CAD build for the part. Positions are in the model's coordinates, mm. A direction names the side the tool comes from. Give positions to 0.01 mm unless a question says otherwise; leave off trailing zeros. Order: outer loops, then holes, each group sorted by start corner. A loop starts at its lowest first (then second) coordinate and runs counter-clockwise, first axis right, second up. Notation, with made-up numbers: (6, -21) -> (53, -21) arc R17 cw to (53, 10) -> close; hole circle Ø2 at (39, 57.5). An arc over 180 degrees is marked (long way). Use one line per item in the form item = value. Start each with the question number.
1) Mould opens along X. For faces 1 (the face through (47.626, 0.805, -46.58)), 2 (the face through (5.15, 0.8, -89.47)), 3 (the face through (28, 1.588, -47)), 4 (the face through (5.557, 0.805, -3.566)) say: pulls with the +X half, pulls with the -X half, needs draft (parallel to the pull), parting line crosses it, or undercut.
2) Probe line 1 (X direction, y = 1.15, z = -5.08); line 2 (Y direction, x = 14.5, z = -10). List the from-to ranges inside material, lowest first.
3) Cut at A-A, the plane z = -5.08. Give the cut face in (x, y).
4) Drop flat-ended pins along their axis: P1, Ø1, axis at x = 44, z = -47, coming from the -Y side; P2, Ø5, axis at x = 52.07, z = -5.08, coming from the +Y side; P3, Ø1.3, axis at y = -1, z = -58.5, coming from the +X side; P4, Ø4, axis at y = -2.5, z = -15, coming from the -X side. Give the stop position or say it passes through.
5) Cut at B-B, the plane x = 22.5. Give the cut face in (y, z).
6) Tool access for faces 5 (the face through (50.52, 0.8, -5.42)), 6 (the face through (5, -1.588, -80)), 7 (the face through (5, -1.588, -58)), 8 (the face through (3.271, -3.131, -75.103)): list every direction of +Z, -Z, +X, -X, +Y, -Y with a clear straight run to the whole face (end or side of a thin tool).
7) Cut at C-C, the plane z = -49.5. Give the cut face in (x, y).
from build123d import *

# Parameters (mm, degrees)
SKETCH1_W           = 57.15
SKETCH1_H           = 92.964
BOSS_EXTRUDE1_DEPTH = 1.5875
SKETCH2_R           = 1.5875
CUT_EXTRUDE1_DEPTH  = 110.137289467
SKETCH3_R           = 4.445
CUT_EXTRUDE2_DEPTH  = 110.137289467
CUT_EXTRUDE3_REACH  = 111.137
SKETCH5_R           = 4.7244
BOSS_EXTRUDE2_DEPTH = 6.35
SKETCH5_3_W         = 4
SKETCH5_3_H         = 4
SKETCH5_3_H_2       = 3
BOSS_EXTRUDE3_DEPTH = 1.5875
SKETCH7_W           = 3
SKETCH7_H           = 1.5
BOSS_EXTRUDE4_DEPTH = 1.5875


with BuildPart() as part:
    # Sketch1 → Boss-Extrude1 (new body)
    with BuildSketch(Plane(origin=(0, 0, 0), x_dir=(1, 0, 0), z_dir=(0, 1, 0))):
        with Locations((28.575, 46.482)):
            Rectangle(SKETCH1_W, SKETCH1_H)
    extrude(amount=BOSS_EXTRUDE1_DEPTH)

    # Sketch2 → Cut-Extrude1 (cut, through all)
    with BuildSketch(Plane(origin=(0, 1.5875, 0), x_dir=(1, 0, 0), z_dir=(0, 1, 0))):
        with Locations(Location((5.08, 87.884, 0), (0, 0, 270))):
            Circle(SKETCH2_R)
        with Locations(Location((52.07, 87.884, 0), (0, 0, 270))):
            Circle(SKETCH2_R)
        with Locations(Location((5.08, 5.08, 0), (0, 0, 270))):
            Circle(SKETCH2_R)
        with Locations(Location((52.07, 5.08, 0), (0, 0, 270))):
            Circle(SKETCH2_R)
    extrude(amount=-CUT_EXTRUDE1_DEPTH, mode=Mode.SUBTRACT)

    # Sketch3 → Cut-Extrude2 (cut, through all)
    with BuildSketch(Plane(origin=(0, 1.5875, 0), x_dir=(1, 0, 0), z_dir=(0, 1, 0))):
        with BuildLine():
            ThreePointArc((56.515, 46.482), (55.213089642, 43.338910358), (52.07, 42.037))
            Line((52.07, 42.037), (57.15, 42.037))
            Line((57.15, 42.037), (57.15, 50.927))
            Line((57.15, 50.927), (52.07, 50.927))
            ThreePointArc((52.07, 50.927), (55.213089642, 49.625089642), (56.515, 46.482))
        make_face()
        with Locations((52.07, 46.482)):
            Circle(SKETCH3_R)
        with Locations((5.08, 46.482)):
            Circle(SKETCH3_R)
        with BuildLine():
            Line((5.08, 50.927), (0, 50.927))
            Line((0, 50.927), (0, 42.037))
            Line((0, 42.037), (5.08, 42.037))
            ThreePointArc((5.08, 42.037), (0.635, 46.482), (5.08, 50.927))
        make_face()
    extrude(amount=-CUT_EXTRUDE2_DEPTH, mode=Mode.SUBTRACT)

    # Sketch4 → Cut-Extrude3 (cut, up to next)
    with BuildSketch(Plane(origin=(0, 1.5875, 0), x_dir=(1, 0, 0), z_dir=(0, 1, 0)), mode=Mode.PRIVATE) as cut_extrude3_sk1:
        with BuildLine():
            ThreePointArc((41.275, 3.175), (43.52006403, 4.10493597), (44.45, 6.35))
            ThreePointArc((44.45, 6.35), (43.52006403, 8.59506403), (41.275, 9.525))
            Line((41.275, 9.525), (41.275, 3.175))
        make_face()
    cut_extrude3_tool1 = extrude(cut_extrude3_sk1.sketch, amount=-CUT_EXTRUDE3_REACH, mode=Mode.PRIVATE) & part.part
    # Sketch4 → Cut-Extrude3 (cut, up to next)
    with BuildSketch(Plane(origin=(0, 1.5875, 0), x_dir=(1, 0, 0), z_dir=(0, 1, 0)), mode=Mode.PRIVATE) as cut_extrude3_sk2:
        with BuildLine():
            Line((41.275, 3.175), (41.275, 9.525))
            ThreePointArc((41.275, 9.525), (39.02993597, 8.59506403), (38.1, 6.35))
            ThreePointArc((38.1, 6.35), (39.02993597, 4.10493597), (41.275, 3.175))
        make_face()
    cut_extrude3_tool2 = extrude(cut_extrude3_sk2.sketch, amount=-CUT_EXTRUDE3_REACH, mode=Mode.PRIVATE) & part.part
    # Sketch4 → Cut-Extrude3 (cut, up to next)
    with BuildSketch(Plane(origin=(0, 1.5875, 0), x_dir=(1, 0, 0), z_dir=(0, 1, 0)), mode=Mode.PRIVATE) as cut_extrude3_sk3:
        with BuildLine():
            ThreePointArc((41.275, 3.175), (43.52006403, 4.10493597), (44.45, 6.35))
            ThreePointArc((44.45, 6.35), (43.52006403, 8.59506403), (41.275, 9.525))
            Line((41.275, 9.525), (41.275, 3.175))
        make_face()
    cut_extrude3_tool3 = extrude(cut_extrude3_sk3.sketch, amount=-CUT_EXTRUDE3_REACH, mode=Mode.PRIVATE) & part.part
    # Sketch4 → Cut-Extrude3 (cut, up to next)
    with BuildSketch(Plane(origin=(0, 1.5875, 0), x_dir=(1, 0, 0), z_dir=(0, 1, 0)), mode=Mode.PRIVATE) as cut_extrude3_sk4:
        with BuildLine():
            Line((41.275, 3.175), (41.275, 9.525))
            ThreePointArc((41.275, 9.525), (39.02993597, 8.59506403), (38.1, 6.35))
            ThreePointArc((38.1, 6.35), (39.02993597, 4.10493597), (41.275, 3.175))
        make_face()
    cut_extrude3_tool4 = extrude(cut_extrude3_sk4.sketch, amount=-CUT_EXTRUDE3_REACH, mode=Mode.PRIVATE) & part.part
    # Sketch4 → Cut-Extrude3 (cut, up to next)
    with BuildSketch(Plane(origin=(0, 1.5875, 0), x_dir=(1, 0, 0), z_dir=(0, 1, 0)), mode=Mode.PRIVATE) as cut_extrude3_sk5:
        with BuildLine():
            Line((41.275, 0), (41.275, 3.175))
            ThreePointArc((41.275, 3.175), (39.02993597, 4.10493597), (38.1, 6.35))
            Line((38.1, 6.35), (38.1, 0))
            Line((38.1, 0), (41.275, 0))
        make_face()
    cut_extrude3_tool5 = extrude(cut_extrude3_sk5.sketch, amount=-CUT_EXTRUDE3_REACH, mode=Mode.PRIVATE) & part.part
    # Sketch4 → Cut-Extrude3 (cut, up to next)
    with BuildSketch(Plane(origin=(0, 1.5875, 0), x_dir=(1, 0, 0), z_dir=(0, 1, 0)), mode=Mode.PRIVATE) as cut_extrude3_sk6:
        with BuildLine():
            Line((44.45, 0), (44.45, 6.35))
            ThreePointArc((44.45, 6.35), (43.52006403, 4.10493597), (41.275, 3.175))
            Line((41.275, 3.175), (41.275, 0))
            Line((41.275, 0), (44.45, 0))
        make_face()
    cut_extrude3_tool6 = extrude(cut_extrude3_sk6.sketch, amount=-CUT_EXTRUDE3_REACH, mode=Mode.PRIVATE) & part.part
    add(cut_extrude3_tool1.solids().sort_by_distance((42.622512, 1.5875, -6.35))[0], mode=Mode.SUBTRACT)
    add(cut_extrude3_tool2.solids().sort_by_distance((39.927488, 1.5875, -6.35))[0], mode=Mode.SUBTRACT)
    add(cut_extrude3_tool3.solids().sort_by_distance((42.622512, 1.5875, -6.35))[0], mode=Mode.SUBTRACT)
    add(cut_extrude3_tool4.solids().sort_by_distance((39.927488, 1.5875, -6.35))[0], mode=Mode.SUBTRACT)
    add(cut_extrude3_tool5.solids().sort_by_distance((39.532316, 1.5875, -1.993291))[0], mode=Mode.SUBTRACT)
    add(cut_extrude3_tool6.solids().sort_by_distance((43.017684, 1.5875, -1.993291))[0], mode=Mode.SUBTRACT)

    # Sketch5 → Boss-Extrude2 (add)
    with BuildSketch(Plane.XZ):
        with Locations(Location((5.08, -70.739, 0), (0, 0, 270))):
            Circle(SKETCH5_R)
    extrude(amount=BOSS_EXTRUDE2_DEPTH)

    # Sketch5<3> → Boss-Extrude3 (add)
    with BuildSketch(Plane.XZ):
        with Locations((5.064710223, -57.987286883)):
            Rectangle(SKETCH5_3_W, SKETCH5_3_H)
        with Locations((5.164801178, -80.177059989)):
            Rectangle(SKETCH5_3_W, SKETCH5_3_H_2)
    extrude(amount=BOSS_EXTRUDE3_DEPTH)

    # Sketch7 → Boss-Extrude4 (add)
    with BuildSketch(Plane(origin=(0, 1.5875, 0), x_dir=(1, 0, 0), z_dir=(0, 1, 0))):
        with Locations((42.270458801, 36.842)):
            Rectangle(SKETCH7_W, SKETCH7_H)
    extrude(amount=BOSS_EXTRUDE4_DEPTH)


solid = part.part
Result:
q1.face_1 = pulls with the +X half
q1.face_2 = undercut
q1.face_3 = needs draft
q1.face_4 = undercut
q2.line_1 = 0 to 3.49, 6.67 to 38.1, 44.45 to 50.48, 53.66 to 57.15
q2.line_2 = 0 to 1.59
q3.outline = (0, 0) -> (3.49, 0) -> (3.49, 1.59) -> (0, 1.59) -> close; (6.67, 0) -> (38.1, 0) -> (38.1, 1.59) -> (6.67, 1.59) -> close; (44.45, 0) -> (50.48, 0) -> (50.48, 1.59) -> (44.45, 1.59) -> close; (53.66, 0) -> (57.15, 0) -> (57.15, 1.59) -> (53.66, 1.59) -> close
q4.P1 = 0
q4.P2 = 1.59
q4.P3 = 7.06
q4.P4 = through
q5.outline = (0, -92.96) -> (1.59, -92.96) -> (1.59, 0) -> (0, 0) -> close
q6.face_5 = +Y, -Y
q6.face_6 = -Z, +X, -X, -Y
q6.face_7 = +Z, +X, -X, -Y
q6.face_8 = -Y
q7.outline = (8.34, 0) -> (48.81, 0) -> (48.81, 1.59) -> (8.34, 1.59) -> close
